```python
from build123d import *

# Parameters (mm, degrees)
SKETCH1_W           = 38.862
SKETCH1_H           = 19.812
BOSS_EXTRUDE1_DEPTH = 0.254
CHAMFER1_SIZE       = 1.27
CHAMFER1_SIZE2      = 0.111110603
CHAMFER2_SIZE       = 1.27
CHAMFER2_SIZE2      = 0.111110603
SKETCH2_W           = 38.862
SKETCH2_H           = 7.112
BOSS_EXTRUDE2_DEPTH = 1.0922
MOVE_FACE1_BY       = 0.3937
MOVE_FACE1_2_BY     = 0.3937
FILLET1_R           = 3.175
FILLET2_R           = 0.381
SKETCH3_W           = 1.27
SKETCH3_H           = 0.642734604
CUT_EXTRUDE1_DEPTH  = 46.780069848
FILLET3_R           = 0.127
FILLET4_R           = 0.127
CUT_EXTRUDE2_DEPTH  = 87.18132095
FILLET5_R           = 1.3716
FILLET6_R           = 1.016
SKETCH5_W           = 2.3876
SKETCH5_H           = 6.1468
CUT_EXTRUDE3_DEPTH  = 87.18132095
FILLET7_R           = 1.1938


# Some blends are built 0.0001 mm under size
with BuildPart() as part:
    # Sketch1 → Boss-Extrude1 (new body)
    with BuildSketch(Plane(origin=(0, 0, 0), x_dir=(1, 0, 0), z_dir=(0, 1, 0))):
        with Locations((-63.262484365, -12.969463084)):
            Rectangle(SKETCH1_W, SKETCH1_H)
    extrude(amount=BOSS_EXTRUDE1_DEPTH)

    # Chamfer1
    chamfer1_edges = [part.edges().sort_by_distance(p)[0] for p in [
        (-63.262484365, 0.254, 22.875463084),
    ]]
    chamfer1_side = [part.faces().sort_by_distance(p)[0] for p in [
        (-63.262484365, 0.254, 12.969463084),
    ]]
    chamfer(chamfer1_edges, length=CHAMFER1_SIZE, length2=CHAMFER1_SIZE2, reference=chamfer1_side[0])

    # Chamfer2
    chamfer2_edges = [part.edges().sort_by_distance(p)[0] for p in [
        (-63.262484365, 0, 22.875463084),
    ]]
    chamfer2_side = [part.faces().sort_by_distance(p)[0] for p in [
        (-63.262484365, 0, 12.969463084),
    ]]
    chamfer(chamfer2_edges, length=CHAMFER2_SIZE, length2=CHAMFER2_SIZE2, reference=chamfer2_side[0])


with BuildPart() as body_2:
    # Sketch2 → Boss-Extrude2 (new body)
    with BuildSketch(Plane(origin=(0, 0.254, 0), x_dir=(-1, 0, 0), z_dir=(0, 1, 0))):
        with Locations((63.262484365, 6.619463084)):
            Rectangle(SKETCH2_W, SKETCH2_H)
    extrude(amount=BOSS_EXTRUDE2_DEPTH)


with BuildPart() as body_2_1:
    # Body-Move/Copy1: moved
    add(body_2.part.moved(Location((0, -0.6731, 0))))

    # Move Face1: a face moved outward by 0.3937
    extrude(body_2_1.faces().sort_by_distance((-82.693484365, 0.127, 6.619463084))[0], amount=MOVE_FACE1_BY, dir=(-1, 0, 0))

    # Move Face1 2: a face moved outward by 0.3937
    extrude(body_2_1.faces().sort_by_distance((-43.831484365, 0.127, 6.619463084))[0], amount=MOVE_FACE1_2_BY, dir=(1, 0, 0))

    # Fillet1
    fillet1_edges = [body_2_1.edges().sort_by_distance(p)[0] for p in [
        (-43.437784365, 0.127, 10.175463084),
        (-83.087184365, 0.127, 10.175463084),
    ]]
    fillet(fillet1_edges, radius=FILLET1_R)


with BuildPart() as part_1:
    add(part.part)

    # Combine1: union body 2
    add(body_2_1.part)

    # Fillet2
    fillet2_edges = [part_1.edges().sort_by_distance(p)[0] for p in [
        (-63.262484365, -0.4191, 3.063463084),
        (-63.262484365, 0.6731, 3.063463084),
    ]]
    fillet(fillet2_edges, radius=FILLET2_R)

    # Sketch3 → Cut-Extrude1 (cut, through all)
    with BuildSketch(Plane(origin=(-43.437784365, 0, 0), x_dir=(0, 0, -1), z_dir=(1, 0, 0))):
        with Locations((-4.706856109, -0.628874986)):
            Rectangle(SKETCH3_W, SKETCH3_H)
        with Locations((-4.706856109, 0.882874986)):
            Rectangle(SKETCH3_W, SKETCH3_H)
    extrude(amount=-CUT_EXTRUDE1_DEPTH, mode=Mode.SUBTRACT)

    # Fillet3
    # the kernel refuses this fillet: 0.127 mm, written as the material it adds along each edge
    with BuildSketch(Plane(origin=(-43.437784365, -0.307507684, 5.341856109), x_dir=(0, 0, -1), z_dir=(-1, 0, 0))) as fillet3_piece_1_section:
        with BuildLine():
            CenterArc((FILLET3_R, FILLET3_R), FILLET3_R, 180, 90)
            Line((0, FILLET3_R), (0, 0))
            Line((0, 0), (FILLET3_R, 0))
        make_face()
    fillet3_piece_1 = extrude(amount=39.6494, mode=Mode.PRIVATE)
    fillet3_piece_1 = split(fillet3_piece_1, bisect_by=Plane(origin=(-63.262484365, -0.4191, 5.312781513), z_dir=(0, 1, 0)), keep=Keep.TOP, mode=Mode.PRIVATE)
    add(fillet3_piece_1)
    with BuildSketch(Plane(origin=(-43.437784365, -0.307507684, 4.071856109), x_dir=(0, -1, 0), z_dir=(-1, 0, 0))) as fillet3_piece_2_section:
        with BuildLine():
            CenterArc((FILLET3_R, FILLET3_R), FILLET3_R, 180, 90)
            Line((0, FILLET3_R), (0, 0))
            Line((0, 0), (FILLET3_R, 0))
        make_face()
    fillet3_piece_2 = extrude(amount=39.6494, mode=Mode.PRIVATE)
    fillet3_piece_2 = split(fillet3_piece_2, bisect_by=Plane(origin=(-63.262484365, -0.4191, 4.100930704), z_dir=(0, 1, 0)), keep=Keep.TOP, mode=Mode.PRIVATE)
    add(fillet3_piece_2)
    with BuildSketch(Plane(origin=(-43.437784365, 0.561507684, 5.341856109), x_dir=(0, 1, 0), z_dir=(-1, 0, 0))) as fillet3_piece_3_section:
        with BuildLine():
            CenterArc((FILLET3_R, FILLET3_R), FILLET3_R, 180, 90)
            Line((0, FILLET3_R), (0, 0))
            Line((0, 0), (FILLET3_R, 0))
        make_face()
    fillet3_piece_3 = extrude(amount=39.6494, mode=Mode.PRIVATE)
    fillet3_piece_3 = split(fillet3_piece_3, bisect_by=Plane(origin=(-63.262484365, 0.6731, 5.312781513), z_dir=(0, -1, 0)), keep=Keep.TOP, mode=Mode.PRIVATE)
    add(fillet3_piece_3)
    with BuildSketch(Plane(origin=(-43.437784365, 0.561507684, 4.071856109), x_dir=(0, 0, 1), z_dir=(-1, 0, 0))) as fillet3_piece_4_section:
        with BuildLine():
            CenterArc((FILLET3_R, FILLET3_R), FILLET3_R, 180, 90)
            Line((0, FILLET3_R), (0, 0))
            Line((0, 0), (FILLET3_R, 0))
        make_face()
    fillet3_piece_4 = extrude(amount=39.6494, mode=Mode.PRIVATE)
    fillet3_piece_4 = split(fillet3_piece_4, bisect_by=Plane(origin=(-63.262484365, 0.6731, 4.100930704), z_dir=(0, -1, 0)), keep=Keep.TOP, mode=Mode.PRIVATE)
    add(fillet3_piece_4)

    # Fillet4
    fillet4_edges = [part_1.edges().sort_by_distance(p)[0] for p in [
        (-63.262484365, -0.4191, 5.340918011),
        (-63.262484365, -0.4191, 4.072794206),
        (-63.262484365, 0.6731, 5.340918011),
        (-63.262484365, 0.6731, 4.072794206),
    ]]
    fillet(fillet4_edges, radius=FILLET4_R)

    # Sketch4 → Cut-Extrude2 (cut, through all)
    with BuildSketch(Plane(origin=(0, 0.254, 0), x_dir=(-1, 0, 0), z_dir=(0, 1, 0))):
        Polygon((82.693484365, 11.699463084), (79.137484365, 11.699463084), (79.137484365, 14.468063084), (84.344362943, 14.468063084), (84.344362943, 11.699463084), align=None)
        Polygon((47.387484365, 14.468063084), (42.180605788, 14.468063084), (42.180605788, 11.699463084), (43.831484365, 11.699463084), (47.387484365, 11.699463084), align=None)
    extrude(amount=-CUT_EXTRUDE2_DEPTH, mode=Mode.SUBTRACT)

    # Fillet5
    fillet5_edges = [part_1.edges().sort_by_distance(p)[0] for p in [
        (-79.137484365, 0.127, 11.699463084),
        (-79.137484365, 0.127, 14.468063084),
        (-47.387484365, 0.127, 14.468063084),
        (-47.387484365, 0.127, 11.699463084),
    ]]
    fillet(fillet5_edges, radius=FILLET5_R)

    # Fillet6
    fillet6_edges = [part_1.edges().sort_by_distance(p)[0] for p in [
        (-82.693484365, 0.127, 11.699463084),
        (-82.693484365, 0.127, 14.468063084),
        (-43.831484365, 0.127, 11.699463084),
        (-43.831484365, 0.127, 14.468063084),
    ]]
    fillet(fillet6_edges, radius=FILLET6_R)

    # Sketch5 → Cut-Extrude3 (cut, through all)
    with BuildSketch(Plane(origin=(0, 0.254, 0), x_dir=(1, 0, 0), z_dir=(0, 1, 0))):
        with Locations((-63.262484365, -13.756863084)):
            Rectangle(SKETCH5_W, SKETCH5_H)
    extrude(amount=-CUT_EXTRUDE3_DEPTH, mode=Mode.SUBTRACT)

    # Fillet7
    fillet7_edges = [part_1.edges().sort_by_distance(p)[0] for p in [
        (-64.456284365, 0.127, 16.830263084),
        (-62.068684365, 0.127, 16.830263084),
        (-62.068684365, 0.127, 10.683463084),
        (-64.456284365, 0.127, 10.683463084),
    ]]
    fillet(fillet7_edges, radius=FILLET7_R - 0.0001)  # a hair under: the kernel refuses the full size


solid = part_1.part
```
Here's how the part is built. I have some questions about the finished solid (model axes, mm). Coordinates: 2 decimals unless noted, no trailing zeros. Order: outer loops, then holes, each group sorted by start corner. A loop starts at its lowest first (then second) coordinate and runs counter-clockwise, first axis right, second up.
Item 1: I need wall thicknesses on probe 1 along Z at (x, y) = (-51.5, -0.1); probe 2 along X at (y, z) = (0.1, 9.75); probe 3 along Z at (x, y) = (-58, 0.6). Which ranges of each line are inside material? Lowest first, please.
Response values:
probe 1: z = 3.07 to 10.18
probe 2: x = -82.69 to -43.83
probe 3: z = 3.22 to 4.11, 5.31 to 10.18
Item 2: If we section it at C-C, the plane z = 19.5: List the corners of the cut face in (x, y) for me, then the cut area to 3 significant figures.
Response values:
outline: (-82.69, 0) - (-43.83, 0) - (-43.83, 0.25) - (-82.69, 0.25) - close
area: 9.87 mm2
Item 3: I'm going to push a flat-ended pin straight in: pin 1 Ø10.5 at (x, z) = (-60, 13.5) entering from -Y. Where does the tip first touch, or does it pass through?
Response values:
pin 1: stops at y = -0.42
Item 4: If we section it at B-B, the plane z = 9.25: List the corners of the cut face in (x, y) for me, then the cut area to 3 significant figures.
Response values:
outline: (-82.69, 0) - (-82.15, 0) - (-82.15, -0.42) - (-44.37, -0.42) - (-44.37, 0) - (-43.83, 0) - (-43.83, 0.25) - (-44.37, 0.25) - (-44.37, 0.67) - (-82.15, 0.67) - (-82.15, 0.25) - (-82.69, 0.25) - close
area: 41.5 mm2
Item 5: Thinking about a two-plate mould opening in Z: for faces 1 (the face through (-63.535, 0.044, 22.108)), 2 (the face through (-63, -0.419, 8)), 3 (the face through (-63, -0.308, 5)), which applies, pulls with the +Z half, pulls with the -Z half, needs draft (parallel to the pull), parting line crosses it, or undercut?
Response values:
face 1: pulls with the +Z half
face 2: needs draft
face 3: undercut
